CAD build for the part. Positions are in the model's coordinates, mm. Face numbers are marked on the shaded views. A direction names the side the tool comes from. Give positions to 0.01 mm unless a question says otherwise; leave off trailing zeros. Order: outer loops, then holes, each group sorted by start corner. A loop starts at its lowest first (then second) coordinate and runs counter-clockwise, first axis right, second up. Notation, with made-up numbers: (-9.75, -4) -> (-0.75, -4) arc R25 cw to (-0.75, 29) -> close; hole circle Ø6 at (48.25, -8). An arc over 180 degrees is marked (long way). Answer as CSV lines item,"result".
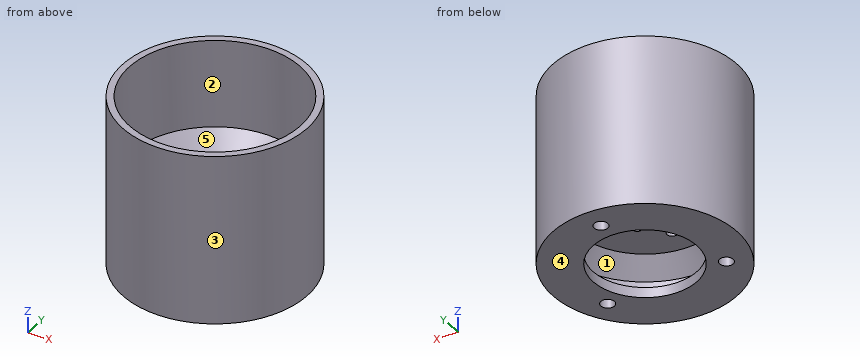
```python
from build123d import *

# Parameters (mm, degrees)
SKETCH2_R          = 2
CUT_EXTRUDE1_DEPTH = 10
SKETCH3_W          = 25.1
SKETCH3_H          = 3
CHAMFER1_SIZE      = 5
SKETCH4_R          = 1.1
SKETCH4_R_2        = 1.5
CUT_EXTRUDE2_DEPTH = 10


with BuildPart() as part:
    # Sketch1 → Revolve1 (revolve)
    with BuildSketch(Plane(origin=(0, 0, 0), x_dir=(1, 0, 0), z_dir=(0, 1, 0))):
        Polygon((15.25, 26.5), (15.25, 23.5), (25.1, 23.5), (25.1, -23.5), (27.1, -23.5), (27.1, 26.5), align=None)
    revolve(axis=Axis((0, 0, -51.288157895), (0, 0, 1)))

    # Sketch2 → Cut-Extrude1 (cut)
    with BuildSketch(Plane(origin=(0, 0, -26.5), x_dir=(-1, 0, 0), z_dir=(0, 0, -1))):
        with Locations((0, 20.25)):
            Circle(SKETCH2_R)
        with Locations((17.537014427, -10.125)):
            Circle(SKETCH2_R)
        with Locations((-17.537014427, -10.125)):
            Circle(SKETCH2_R)
    extrude(amount=-CUT_EXTRUDE1_DEPTH, mode=Mode.SUBTRACT)

    # Sketch3 → Revolve2 (revolve)
    with BuildSketch(Plane(origin=(0, 0, 0), x_dir=(1, 0, 0), z_dir=(0, 1, 0))):
        with Locations((12.55, 8.8)):
            Rectangle(SKETCH3_W, SKETCH3_H)
    revolve(axis=Axis((0, 0, -51.288157895), (0, 0, 1)))

    # Chamfer1
    chamfer1_edges = [part.edges().sort_by_distance(p)[0] for p in [
        (-25.1, 0, -7.3),
        (-25.1, 0, -10.3),
    ]]
    chamfer(chamfer1_edges, length=CHAMFER1_SIZE)

    # Sketch4 → Cut-Extrude2 (cut)
    with BuildSketch(Plane(origin=(0, 0, -10.3), x_dir=(-1, 0, 0), z_dir=(0, 0, -1))):
        with Locations((-6.363961031, 6.363961031)):
            Circle(SKETCH4_R)
        with Locations((6.363961031, 6.363961031)):
            Circle(SKETCH4_R)
        with Locations((6.363961031, -6.363961031)):
            Circle(SKETCH4_R)
        with Locations((-6.363961031, -6.363961031)):
            Circle(SKETCH4_R)
        with Locations((0, 12.5)):
            Circle(SKETCH4_R_2)
        with Locations((0, -12.5)):
            Circle(SKETCH4_R_2)
        with BuildLine():
            Line((-6.05, 3.619392214), (-6.05, -3.619392214))
            ThreePointArc((-6.05, -3.619392214), (0, -7.05), (6.05, -3.619392214))
            Line((6.05, -3.619392214), (6.05, 3.619392214))
            ThreePointArc((6.05, 3.619392214), (0, 7.05), (-6.05, 3.619392214))
        make_face()
    extrude(amount=-CUT_EXTRUDE2_DEPTH, mode=Mode.SUBTRACT)


solid = part.part
```
1) Pin check, flat tips, straight feed: P1, Ø1.5, axis at x = 0, y = 14.5, coming from the +Z side; P2, Ø2, axis at y = 6.5, z = -14.5, coming from the -X side; P3, Ø6, axis at y = 17.5, z = 8.5, coming from the -X side; P4, Ø2.5, axis at x = 0, y = -12.5, coming from the +Z side. Stop position of each tip, or through.
Data:
P1,"stops at z = -7.3"
P2,"stops at x = -26.54"
P3,"stops at x = -22.89"
P4,"passes through"
2) Which spindle directions (+Z, -Z, +X, -X, +Y, -Y) get a long thin tool onto all of the face, cutting with end or side? Do the marked faces 1 and 2. Say none if no direction does.
Data:
face 1,"none"
face 2,"+Z"
3) Band-saw the part on A-A, the plane y = 0. Write the cut outline in (x, z), then the cut area to 3 significant figures.
Data:
outline,"(-27.1, -26.5) -> (-15.25, -26.5) -> (-15.25, -23.5) -> (-25.1, -23.5) -> (-25.1, -15.3) -> (-20.1, -10.3) -> (-6.05, -10.3) -> (-6.05, -7.3) -> (-20.1, -7.3) -> (-25.1, -2.3) -> (-25.1, 23.5) -> (-27.1, 23.5) -> close; (6.05, -10.3) -> (20.1, -10.3) -> (25.1, -15.3) -> (25.1, -23.5) -> (15.25, -23.5) -> (15.25, -26.5) -> (27.1, -26.5) -> (27.1, 23.5) -> (25.1, 23.5) -> (25.1, -2.3) -> (20.1, -7.3) -> (6.05, -7.3) -> close"
area,"423 mm2"
4) Wall check: line 1 along Y through (x, z) = (0, -25.7); line 2 along Y through (x, z) = (0, -9.25); line 3 along Y through (x, z) = (0, 14.75). Give the ranges that are in metal, low to high. Write a range as [from, to].
Data:
line 1,"y = [-27.1, -15.25], [15.25, 18.25], [22.25, 27.1]"
line 2,"y = [-27.1, -14], [-11, -7.05], [7.05, 11], [14, 27.1]"
line 3,"y = [-27.1, -25.1], [25.1, 27.1]"
5) Pull direction X, two halves, no side cores. Call the marked faces 3, 4 and 5: pulls with the +X half, pulls with the -X half, needs draft (parallel to the pull), parting line crosses it, or undercut.
Data:
face 3,"parting line crosses it"
face 4,"needs draft"
face 5,"undercut"
6) Band-saw the part on B-B, the plane x = 0. Give the number of separate pieces and of enclosed holes in the cut face, then the cut area to 3 significant figures.
Data:
separate pieces,"5"
enclosed holes,"0"
area,"387 mm2"
7) Band-saw the part on C-C, the plane z = -4.5. Write the cut outline in (x, y).
Data:
outline,"circle Ø54.2 at (0, 0); hole circle Ø45.8 at (0, 0)"
8) Band-saw the part on D-D, the plane z = -17.5. Write the cut outline in (x, y).
Data:
outline,"circle Ø54.2 at (0, 0); hole circle Ø50.2 at (0, 0)"
